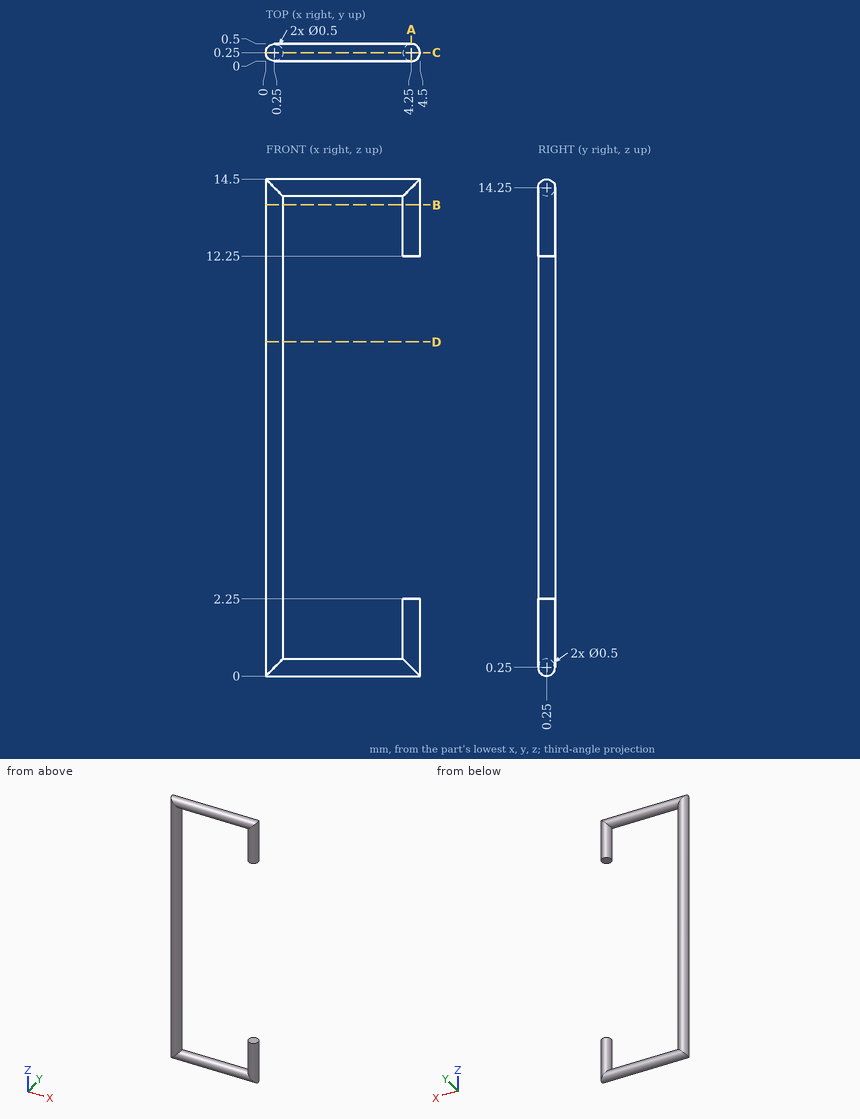
Verification items for this drawing (mm, ordinates from the low corner). Round coordinates to 2 decimals unless told otherwise and drop trailing zeros. Write each loop counter-clockwise with the first axis right and the second up, starting at its lowest first coordinate (ties: lowest second). Pieces come first, ordered by that corner, then holes. Notation, with made-up numbers: M -26,20 L 16,20 A36 ccw 16,57 Z; hole C 28.5,-33 d6. An arc over 180 degrees is marked long. Write item = value, one per line. Start each with the question number.
1. Section check D-D, the plane z = 9.75. Record the cut outline in (x, y).
2. Section check A-A, the plane x = 4.25. Record the cut outline in (y, z).
3. Section check B-B, the plane z = 13.75. Record the cut outline in (x, y).
4. Scan lines: line 1 (Z direction, x = 2.6, y = 0.25); line 2 (Z direction, x = 4.15, y = 0.25); line 3 (X direction, y = 0.4, z = 2). Record each from-to range of solid material in increasing order. Write a range as [from, to].
5. Section check C-C, the plane y = 0.25. Record the cut outline in (x, z), then the cut area to 3 significant figures.
Results found:
q1.outline = C 0.25,0.25 d0.5
q2.outline = M 0,0.25 A0.25 ccw 0.5,0.25 L 0.5,2.25 L 0,2.25 Z; M 0,12.25 L 0.5,12.25 L 0.5,14.25 A0.25 ccw 0,14.25 Z
q3.outline = C 0.25,0.25 d0.5; C 4.25,0.25 d0.5
q4.line_1 = [0, 0.5], [14, 14.5]
q4.line_2 = [0, 2.25], [12.25, 14.5]
q4.line_3 = [0.05, 0.45], [4.05, 4.45]
q5.outline = M 0,0 L 4.5,0 L 4.5,2.25 L 4,2.25 L 4,0.5 L 0.5,0.5 L 0.5,14 L 4,14 L 4,12.25 L 4.5,12.25 L 4.5,14.5 L 0,14.5 Z
q5.area = 13.0 mm^2
